Part model, mm, in its own coordinate system. Face numbers are marked on the shaded views. A direction names the side the tool comes from. Give positions to 0.01 mm unless a question says otherwise; leave off trailing zeros. Order: outer loops, then holes, each group sorted by start corner. A loop starts at its lowest first (then second) coordinate and runs counter-clockwise, first axis right, second up. Notation, with made-up numbers: (84.25, 70.5) -> (118.25, 70.5) arc R24 ccw to (118.25, 83.5) -> close; hole circle Ø10 at (-36.5, -14.75). An arc over 180 degrees is marked (long way). Write item = value, one per line. Start each with the question number.
Item 1: Band-saw the part on D-D on x = -99. Write the cut outline in (y, z) (3 decimals), plus the area to 3 significant figures.
Item 2: Tool access for the marked faces 5 and 6: list every direction of +Z, -Z, +X, -X, +Y, -Y with a clear straight run to the whole face (end or side of a thin tool).
Item 3: Band-saw the part on C-C on z = 23. Write the cut outline in (x, y) (3 decimals).
Item 4: Band-saw the part on B-B on x = -88.5. Write the cut outline in (y, z) (3 decimals), plus the area to 3 significant figures.
Item 5: Pull direction X, two halves, no side cores. Call the marked faces 1, 2, 3 and 4: +X half, -X half, draft (parallel to the pull), parting line (faces both ways), or undercut.
Item 6: Flat gauge pin, fed straight in: P1, Ø8, axis at x = -102.5, y = 55.5, coming from the -Z side. Where does the tip first touch, or does it go through?
Item 7: Band-saw the part on A-A on y = 33. Write the cut outline in (x, z).
Item 8: Drill centre lines: line 1 along Y through (x, z) = (-86, 3.5) (3 decimals); line 2 along X through (y, z) = (-65, 31); line 3 along Y through (x, z) = (-102, 30.5) (3 decimals). Where is each one in solid material? Low to high.
```python
from build123d import *

# Parameters (mm, degrees)
F1_DEPTH = 50.8
F2_W     = 20.828
F2_H     = 38.1
F3_DEPTH = 50.8
F4_W     = 22.225
F4_H     = 53.975
F5_DEPTH = 50.8
F6_R     = 8.89
F7_R     = 2.54
F8_W     = 276.807827
F8_H     = 218.873116
F9_DEPTH = 50.8


with BuildPart() as f1:
    # F0 (on Top) → F1 (new body)
    with BuildSketch(Plane.XY):
        with BuildLine():
            ThreePointArc((-111.331622, 89), (-115.642145, 87.214523), (-117.427622, 82.904))
            Line((-117.427622, 82.904), (-117.427622, -82.904))
            ThreePointArc((-117.427622, -82.904), (-115.642145, -87.214523), (-111.331622, -89))
            Line((-111.331622, -89), (111.331622, -89))
            ThreePointArc((111.331622, -89), (115.642145, -87.214523), (117.427622, -82.904))
            Line((117.427622, -82.904), (117.427622, 82.904))
            ThreePointArc((117.427622, 82.904), (115.642145, 87.214523), (111.331622, 89))
            Line((111.331622, 89), (-111.331622, 89))
        make_face()
        with BuildLine():
            ThreePointArc((-60.918022, -10.802655), (-61.609639, -0.559986), (-60.913995, 9.68241))
            Line((-60.913995, 9.68241), (-55.212554, 14.261207))
            ThreePointArc((-55.212554, 14.261207), (-45.748511, 39.77658), (-28.391702, 60.737103))
            Line((-28.391702, 60.737103), (-27.407633, 67.742944))
            ThreePointArc((-27.407633, 67.742944), (-18.790824, 73.526894), (-9.485241, 78.121416))
            Line((-9.485241, 78.121416), (-2.738388, 75.428307))
            ThreePointArc((-2.738388, 75.428307), (24.098624, 80.048241), (50.935831, 75.42944))
            Line((50.935831, 75.42944), (57.610091, 78.186609))
            ThreePointArc((57.610091, 78.186609), (66.892407, 73.605247), (75.516596, 67.880422))
            Line((75.516596, 67.880422), (76.520517, 60.753405))
            ThreePointArc((76.520517, 60.753405), (79.783196, 57.954312), (82.843276, 54.935057))
            ThreePointArc((82.843276, 54.935057), (104.449894, 47.071779), (100.407804, 24.436881))
            ThreePointArc((100.407804, 24.436881), (101.514269, 20.155202), (102.319921, 15.806873))
            Line((102.319921, 15.806873), (108.049072, 10.873495))
            ThreePointArc((108.049072, 10.873495), (108.709842, 0.589153), (108.105719, -9.698672))
            Line((108.105719, -9.698672), (102.348457, -13.775574))
            ThreePointArc((102.348457, -13.775574), (92.855411, -39.306001), (75.46826, -60.272823))
            Line((75.46826, -60.272823), (74.544008, -67.341163))
            ThreePointArc((74.544008, -67.341163), (66.082602, -73.324939), (56.891661, -78.113213))
            Line((56.891661, -78.113213), (50.250983, -75.428069))
            ThreePointArc((50.250983, -75.428069), (23.341097, -80.124901), (-3.581639, -75.502299))
            Line((-3.581639, -75.502299), (-10.28992, -78.054152))
            ThreePointArc((-10.28992, -78.054152), (-19.562426, -73.562391), (-28.115124, -67.817248))
            Line((-28.115124, -67.817248), (-29.074377, -60.66791))
            ThreePointArc((-29.074377, -60.66791), (-32.330068, -57.869325), (-35.398386, -54.86649))
            ThreePointArc((-35.398386, -54.86649), (-59.811696, -48.379935), (-53.325141, -23.966625))
            ThreePointArc((-53.325141, -23.966625), (-54.434448, -19.687429), (-55.222977, -15.337682))
            Line((-55.222977, -15.337682), (-60.918022, -10.802655))
        make_face(mode=Mode.SUBTRACT)
    extrude(amount=F1_DEPTH)

    # F2 (on face) → F3 (cut)
    with BuildSketch(Plane.XY.offset(50.8)):
        with Locations((-94.313622, -57.25)):
            Rectangle(F2_W, F2_H)
        with Locations((-94.313622, -6.45)):
            Rectangle(F2_W, F2_H)
    extrude(amount=-F3_DEPTH, mode=Mode.SUBTRACT)

    # F4 (on face) → F5 (cut)
    with BuildSketch(Plane.XY.offset(50.8)):
        with Locations((-93.615122, 49.3125)):
            Rectangle(F4_W, F4_H)
    extrude(amount=-F5_DEPTH, mode=Mode.SUBTRACT)

    # F6
    f6_edges = [f1.edges().sort_by_distance(p)[0] for p in [
        (-104.727622, 12.6, 25.4),
        (-104.727622, -38.2, 25.4),
        (-104.727622, -25.5, 25.4),
        (-104.727622, -76.3, 25.4),
    ]]
    fillet(f6_edges, radius=F6_R)

    # F7
    f7_edges = [f1.edges().sort_by_distance(p)[0] for p in [
        (-82.502622, 76.3, 25.4),
        (-104.727622, 76.3, 25.4),
        (-82.502622, 22.325, 25.4),
        (-104.727622, 22.325, 25.4),
    ]]
    fillet(f7_edges, radius=F7_R)

    # F8 (on face) → F9 (cut)
    with BuildSketch(Plane.XY.offset(50.8)):
        with Locations((67.585292, -20.436558)):
            Rectangle(F8_W, F8_H)
    extrude(amount=-F9_DEPTH, mode=Mode.SUBTRACT)


solid = f1.part
```
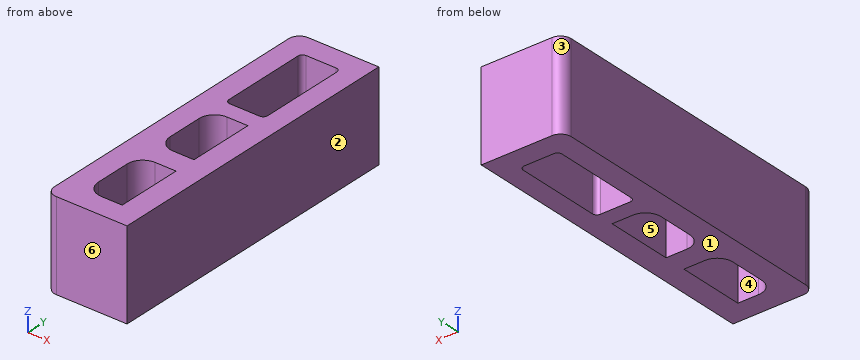
Values found:
q1.outline = (-89, 0) -> (-75.719, 0) -> (-75.719, 50.8) -> (-89, 50.8) -> close; (-38.781, 0) -> (-24.919, 0) -> (-24.919, 50.8) -> (-38.781, 50.8) -> close; (12.019, 0) -> (22.325, 0) -> (22.325, 50.8) -> (12.019, 50.8) -> close; (76.3, 0) -> (89, 0) -> (89, 50.8) -> (76.3, 50.8) -> close
q1.area = 2,550 mm^2
q2.face_5 = +Z, -Z
q2.face_6 = +Z, -Z, +X, -X, -Y
q3.outline = (-117.428, -82.904) arc R6.096 ccw to (-111.332, -89) -> (-70.819, -89) -> (-70.819, 89) -> (-111.332, 89) arc R6.096 ccw to (-117.428, 82.904) -> close; hole (-104.728, -67.41) arc R8.89 ccw to (-95.838, -76.3) -> (-83.9, -76.3) -> (-83.9, -38.2) -> (-95.838, -38.2) arc R8.89 ccw to (-104.728, -47.09) -> close; hole (-104.728, -16.61) arc R8.89 ccw to (-95.838, -25.5) -> (-83.9, -25.5) -> (-83.9, 12.6) -> (-95.838, 12.6) arc R8.89 ccw to (-104.728, 3.71) -> close; hole (-104.728, 24.865) arc R2.54 ccw to (-102.188, 22.325) -> (-85.043, 22.325) arc R2.54 ccw to (-82.503, 24.865) -> (-82.503, 73.76) arc R2.54 ccw to (-85.043, 76.3) -> (-102.188, 76.3) arc R2.54 ccw to (-104.728, 73.76) -> close
q4.outline = (-89, 0) -> (-76.3, 0) -> (-76.3, 50.8) -> (-89, 50.8) -> close; (-38.2, 0) -> (-25.5, 0) -> (-25.5, 50.8) -> (-38.2, 50.8) -> close; (12.6, 0) -> (22.325, 0) -> (22.325, 50.8) -> (12.6, 50.8) -> close; (76.3, 0) -> (89, 0) -> (89, 50.8) -> (76.3, 50.8) -> close
q4.area = 2,430 mm^2
q5.face_1 = draft
q5.face_2 = +X half
q5.face_3 = -X half
q5.face_4 = undercut
q6.P1 = 0
q7.outline = (-117.43, 0) -> (-104.73, 0) -> (-104.73, 50.8) -> (-117.43, 50.8) -> close; (-82.5, 0) -> (-70.82, 0) -> (-70.82, 50.8) -> (-82.5, 50.8) -> close
q8.line_1 = -89 to -76.3, -38.2 to -25.5, 12.6 to 22.325, 76.3 to 89
q8.line_2 = -117.43 to -104.73, -83.9 to -70.82
q8.line_3 = -89 to -73.818, -40.682 to -23.018, 10.118 to 22.325, 76.3 to 89
